Can you work these out from the model? Positions are in its coordinate system, mm. A direction names the side the tool comes from. Give positions to 0.01 mm unless a question says otherwise; leave off trailing zeros. Order: outer loops, then holes, each group sorted by start corner. A loop starts at its lowest first (then second) coordinate and runs counter-clockwise, first axis right, second up. Notation, with made-up numbers: M 0,58.5 L 20,58.5 A22 ccw 20,68.5 Z; hole C -14.5,-29.75 d2. An arc over 180 degrees is marked long. Use a Markdown table: item, result. Add a question column.
from build123d import *

# Parameters (mm, degrees)
F1_DEPTH   = 25.4
F4_D       = 3.175
F4_ON_F3_D = 3.175


with BuildPart() as f1:
    # F0 (on Front) → F1 (new body)
    with BuildSketch(Plane.XZ):
        Polygon((0, 25.4), (0, 0), (25.4, 0), (25.4, 2.54), (2.54, 2.54), (2.54, 25.4), align=None)
    extrude(amount=F1_DEPTH)

    # F4 (through all)
    with Locations(Plane.YZ.offset(2.54)):
        with Locations((-12.7, 12.7)):
            Hole(F4_D / 2)

    # F4 on F3 (through all)
    with Locations(Plane.XY.offset(2.54)):
        with Locations((12.7, -12.7)):
            Hole(F4_ON_F3_D / 2)


solid = f1.part
1. I need wall thicknesses on L1, parallel to Z at x = 0.95, y = -12.7; L2, parallel to Z at x = 9, y = -1. Which ranges of each line are inside material? Lowest first, please. Write a range as [from, to].
2. Will these pins go through, and if not, where does the flat tip stop? pin 1 (10 mm diameter, centred on x = 15, y = -9, fed in from -Z); pin 2 (2 mm diameter, centred on y = -7.5, z = 20.5, fed in from +X); pin 3 (1.5 mm diameter, centred on x = 13.5, y = -18.5, fed in from +Z).
3. We'd pull the mould along Y, two halves only. Please class faces 1 (the face through (7, 0, 2)), 2 (the face through (1.252, -14.214, 13.177)), 3 (the face through (11.186, -12.223, 1.252)), 4 (the face through (17, -13, 2.54)): +Y half, -Y half, draft (parallel to the pull), parting line (faces both ways), or undercut.
4. On a 3-axis mill with a long thin cutter (end or side, diameter ignored), from which of +Z, -Z, +X, -X, +Y, -Y can I reach the whole of each face in a straight line? I mean faces 5 (the face through (25.4, -13, 1)), 6 (the face through (2.54, -13, 16)). Say none if no direction works.
5. If we section it at D-D, the plane z = 23.5: List the corners of the cut face in (x, y) for me, then the cut area to 3 significant figures.
6. If we section it at A-A, the plane x = 12.7: List the corners of the cut face in (y, z) for me.
7. If we section it at C-C, the plane y = -12.7: List the corners of the cut face in (x, z) for me, then the cut area to 3 significant figures.
8. If we section it at B-B, the plane z = 12.7: List the corners of the cut face in (x, y) for me, then the cut area to 3 significant figures.
Geometry results:
| question | item | result |
|---|---|---|
| 1 | L1 | z = [0, 11.11], [14.29, 25.4] |
| 1 | L2 | z = [0, 2.54] |
| 2 | pin 1 | stops at z = 0 |
| 2 | pin 2 | stops at x = 2.54 |
| 2 | pin 3 | stops at z = 2.54 |
| 3 | face 1 | +Y half |
| 3 | face 2 | undercut |
| 3 | face 3 | undercut |
| 3 | face 4 | draft |
| 4 | face 5 | +Z, -Z, +X, +Y, -Y |
| 4 | face 6 | +Z, +X, +Y, -Y |
| 5 | outline | M 0,-25.4 L 2.54,-25.4 L 2.54,0 L 0,0 Z |
| 5 | area | 64.5 mm^2 |
| 6 | outline | M -25.4,0 L -14.29,0 L -14.29,2.54 L -25.4,2.54 Z; M -11.11,0 L 0,0 L 0,2.54 L -11.11,2.54 Z |
| 7 | outline | M 0,0 L 11.11,0 L 11.11,2.54 L 2.54,2.54 L 2.54,11.11 L 0,11.11 Z; M 0,14.29 L 2.54,14.29 L 2.54,25.4 L 0,25.4 Z; M 14.29,0 L 25.4,0 L 25.4,2.54 L 14.29,2.54 Z |
| 7 | area | 106 mm^2 |
| 8 | outline | M 0,-25.4 L 2.54,-25.4 L 2.54,-14.29 L 0,-14.29 Z; M 0,-11.11 L 2.54,-11.11 L 2.54,0 L 0,0 Z |
| 8 | area | 56.5 mm^2 |
